Geometry check sheet. Reference: the model listing, model coordinates, mm. A direction names the side the tool comes from. Round coordinates to 2 decimals unless told otherwise and drop trailing zeros. Order: outer loops, then holes, each group sorted by start corner. A loop starts at its lowest first (then second) coordinate and runs counter-clockwise, first axis right, second up. Notation, with made-up numbers: (33.5, 2) -> (67.5, 2) arc R15 cw to (67.5, 7) -> close; hole circle Ø10 at (58.25, 21). An arc over 180 degrees is marked (long way). Use a Markdown table: item, result. Add a question column.
Item 1: Gauge pin test, flat ends, axial feed: pin 1 Ø4.5 at (x, y) = (-9.525, 0) entering from -Z; pin 2 Ø6.5 at (x, y) = (0, 0) entering from -Z. Record the tip position at first contact, or that the pin passes through.
Item 2: Set-up check for faces 5 (the cylindrical face through (-5.158, 3.955, 0.74)), 6 (the flat face through (0, -6, 2)): record each of +Z, -Z, +X, -X, +Y, -Y from which the full face is reachable in a straight line by a thin tool's end or side.
Item 3: Sectioned sample at D-D, the plane z = 0.35. Record the cut outline in (x, y) (3 decimals).
Item 4: Material ranges on probe 1 along Y at (x, z) = (0, 1.85); probe 2 along Y at (x, z) = (0, 0.8); probe 3 along X at (y, z) = (-1, 1) (3 decimals), recorded low to high. Write a range as [from, to].
Item 5: Sectioned sample at C-C, the plane x = 10.5. Record the cut outline in (y, z).
Item 6: Sectioned sample at A-A, the plane y = 0. Record the cut outline in (x, z) (3 decimals), and give its area (3 significant figures).
Item 7: Sectioned sample at B-B, the plane x = 0. Record the cut outline in (y, z).
Item 8: Mould release check, pull along Y, two halves, no side actions. Record for faces 1 (the flat face through (3, -6, 0)), 2 (the cylindrical face through (-1.19, 5.37, 1.75)), 3 (the cylindrical face through (6.691, 12.864, 0.986)), 4 (the flat face through (-5, 3, 1.5)): pulls with the +Y half, pulls with the -Y half, needs draft (parallel to the pull), parting line crosses it, or undercut.
Autodesk Inventor part; units mm, degrees
ref_plane "YZ Plane" through (0, 0, 0) normal (1, 0, 0) x (0, 1, 0)
ref_plane "XZ Plane" through (0, 0, 0) normal (0, 1, 0) x (-1, 0, 0)
ref_plane "XY Plane" through (0, 0, 0) normal (0, 0, 1) x (1, 0, 0)
sketch "Skizze1" plane through (0, 0, 0) normal (0, 0, 1) x (1, 0, 0)
  circle A0 centre (0, 0) radius 14.5
  circle A1 centre (0, 0) radius 9.525 construction
  circle A2 centre (0, 0) radius 5.5
  circle A3 centre (0, 0) radius 6.5
  line L0 (-9.525, 0) -> (9.525, 0) construction
  circle A4 centre (0, 0) radius 10.45 construction
  line L1 (0, 0) -> (0, 10.45) construction
  point P0 (-9.05, -5.225)
  point P1 (9.05, -5.225)
  dimension "d15" = 20.9
  dimension "d0" = 29
  dimension "d1" = 19.05
  dimension "d2" = 11
  dimension "d3" = 13
  dimension "d18" = 360
extrude "Extrusion1" add sketch "Skizze1" along normal blind 2 contours A0 | A3
extrude "Extrusion2" cut sketch "Skizze1" along normal blind 1.5 contours A3
hole "Bohrung1" at (-9.525, 0, 0) at (9.525, 0, 0) direction (0, 0, 1) diameter 2.9 end through all
properties part number "Sensor_AbstandFlansch"
Found:
| question | item | result |
|---|---|---|
| 1 | pin 1 | stops at z = 0 |
| 1 | pin 2 | passes through |
| 2 | face 5 | -Z |
| 2 | face 6 | +Z, +X, -X, +Y, -Y |
| 3 | outline | circle Ø29 at (0, 0); hole circle Ø2.9 at (-9.525, 0); hole circle Ø13 at (0, 0); hole circle Ø2.9 at (9.525, 0) |
| 4 | probe 1 | y = [-14.5, -5.5], [5.5, 14.5] |
| 4 | probe 2 | y = [-14.5, -6.5], [6.5, 14.5] |
| 4 | probe 3 | x = [-14.465, -10.575], [-8.475, -6.423], [6.423, 8.475], [10.575, 14.465] |
| 5 | outline | (-10, 0) -> (-1.07, 0) -> (-1.07, 2) -> (-10, 2) -> close; (1.07, 0) -> (10, 0) -> (10, 2) -> (1.07, 2) -> close |
| 6 | outline | (-14.5, 0) -> (-10.975, 0) -> (-10.975, 2) -> (-14.5, 2) -> close; (-8.075, 0) -> (-6.5, 0) -> (-6.5, 1.5) -> (-5.5, 1.5) -> (-5.5, 2) -> (-8.075, 2) -> close; (5.5, 1.5) -> (6.5, 1.5) -> (6.5, 0) -> (8.075, 0) -> (8.075, 2) -> (5.5, 2) -> close; (10.975, 0) -> (14.5, 0) -> (14.5, 2) -> (10.975, 2) -> close |
| 6 | area | 21.4 mm2 |
| 7 | outline | (-14.5, 0) -> (-6.5, 0) -> (-6.5, 1.5) -> (-5.5, 1.5) -> (-5.5, 2) -> (-14.5, 2) -> close; (5.5, 1.5) -> (6.5, 1.5) -> (6.5, 0) -> (14.5, 0) -> (14.5, 2) -> (5.5, 2) -> close |
| 8 | face 1 | needs draft |
| 8 | face 2 | undercut |
| 8 | face 3 | parting line crosses it |
| 8 | face 4 | undercut |
